```python
from build123d import *

# Parameters (mm, degrees)
PAD_DEPTH    = 39.3
SKETCH001_R  = 1.5
POCKET_DEPTH = 4.5
SKETCH002_R  = 11
PAD001_DEPTH = 2
SKETCH003_R  = 2.5
PAD002_DEPTH = 23.5


with BuildPart() as part:
    # Sketch → Pad (new body)
    with BuildSketch(Plane.XY):
        Polygon((-16.15, 21.15), (-21.15, 16.15), (-21.15, -16.15), (-16.15, -21.15), (16.15, -21.15), (21.15, -16.15), (21.15, 16.15), (16.15, 21.15), align=None)
    extrude(amount=PAD_DEPTH)

    # Sketch001 → Pocket (cut)
    with BuildSketch(Plane.XY):
        with Locations((-15.5, 15.5)):
            Circle(SKETCH001_R)
        with Locations((-15.5, -15.5)):
            Circle(SKETCH001_R)
        with Locations((15.5, -15.5)):
            Circle(SKETCH001_R)
        with Locations((15.5, 15.5)):
            Circle(SKETCH001_R)
    extrude(amount=POCKET_DEPTH, mode=Mode.SUBTRACT)

    # Sketch002 → Pad001 (join)
    with BuildSketch(Plane.XY):
        Circle(SKETCH002_R)
    extrude(amount=-PAD001_DEPTH)

    # Sketch003 → Pad002 (join)
    with BuildSketch(Plane.XY):
        Circle(SKETCH003_R)
    extrude(amount=-PAD002_DEPTH)


solid = part.part
```
The listing builds one solid part. Answer for the finished solid, in the listing's coordinates (mm). A direction names the side the tool comes from. Round coordinates to 2 decimals unless told otherwise and drop trailing zeros. Write each loop counter-clockwise with the first axis right and the second up, starting at its lowest first coordinate (ties: lowest second). Pieces come first, ordered by that corner, then holes. Notation, with made-up numbers: (83, -6) -> (102, -6) arc R16 ccw to (102, 5) -> close; hole circle Ø1 at (-2, 53.5). An arc over 180 degrees is marked (long way). Answer as a JSON object with one key per item and string values. Group by question number.
Q1. Straight lines are drawn through the part: line 1 along Y through (x, z) = (15.5, 1.5); line 2 along X through (y, z) = (15, 2). For each, find the intervals that lie inside material, in ascending order.
Q2. Section A-A (z = 32) is taken. Write down the section's boundary in (x, y), plus the area to 3 significant figures.
Q3. Section D-D (x = -6) is taken. Write down the section's boundary in (y, z), plus the area to 3 significant figures.
Q4. Which of the six approach directions +Z, -Z, +X, -X, +Y, -Y give full straight-line access (tool end or side, diameter ignored) to faces 1 (the face through (0, 0, -23.5)), 2 (the face through (14, -15.43, 2.22))?
Q5. Section B-B (x = 0) is taken. Write down the section's boundary in (y, z).
Q6. Determine the mould class of faces 3 (the face through (15, 16, 4.5)), 4 (the face through (0, -21.15, 19)), 5 (the face through (-3, 0, -2)) for opening direction Y: pulls with the +Y half, pulls with the -Y half, needs draft (parallel to the pull), parting line crosses it, or undercut.
Q7. Each of these flat-tipped pins is pushed along its axis until it touches: pin 1 Ø8 at (x, y) = (-3, -7) entering from -Z; pin 2 Ø3.5 at (x, y) = (15.5, 15.5) entering from -Z; pin 3 Ø2.5 at (x, y) = (-15.5, 15.5) entering from -Z; pin 4 Ø6.5 at (x, y) = (-3.5, 4) entering from -Z. Where does it stop, or does it pass through?
Check values:
{
 "1": {"line 1": "-21.15 to -17, -14 to 14, 17 to 21.15", "line 2": "-21.15 to -16.91, -14.09 to 14.09, 16.91 to 21.15"},
 "2": {"outline": "(-21.15, -16.15) -> (-16.15, -21.15) -> (16.15, -21.15) -> (21.15, -16.15) -> (21.15, 16.15) -> (16.15, 21.15) -> (-16.15, 21.15) -> (-21.15, 16.15) -> close", "area": "1,740 mm^2"},
 "3": {"outline": "(-21.15, 0) -> (-9.22, 0) -> (-9.22, -2) -> (9.22, -2) -> (9.22, 0) -> (21.15, 0) -> (21.15, 39.3) -> (-21.15, 39.3) -> close", "area": "1,700 mm^2"},
 "4": {"face 1": "-Z, +X, -X, +Y, -Y", "face 2": "-Z"},
 "5": {"outline": "(-21.15, 0) -> (-11, 0) -> (-11, -2) -> (-2.5, -2) -> (-2.5, -23.5) -> (2.5, -23.5) -> (2.5, -2) -> (11, -2) -> (11, 0) -> (21.15, 0) -> (21.15, 39.3) -> (-21.15, 39.3) -> close"},
 "6": {"face 3": "undercut", "face 4": "pulls with the -Y half", "face 5": "needs draft"},
 "7": {"pin 1": "z = -2", "pin 2": "z = 0", "pin 3": "z = 4.5", "pin 4": "z = -23.5"}
}
